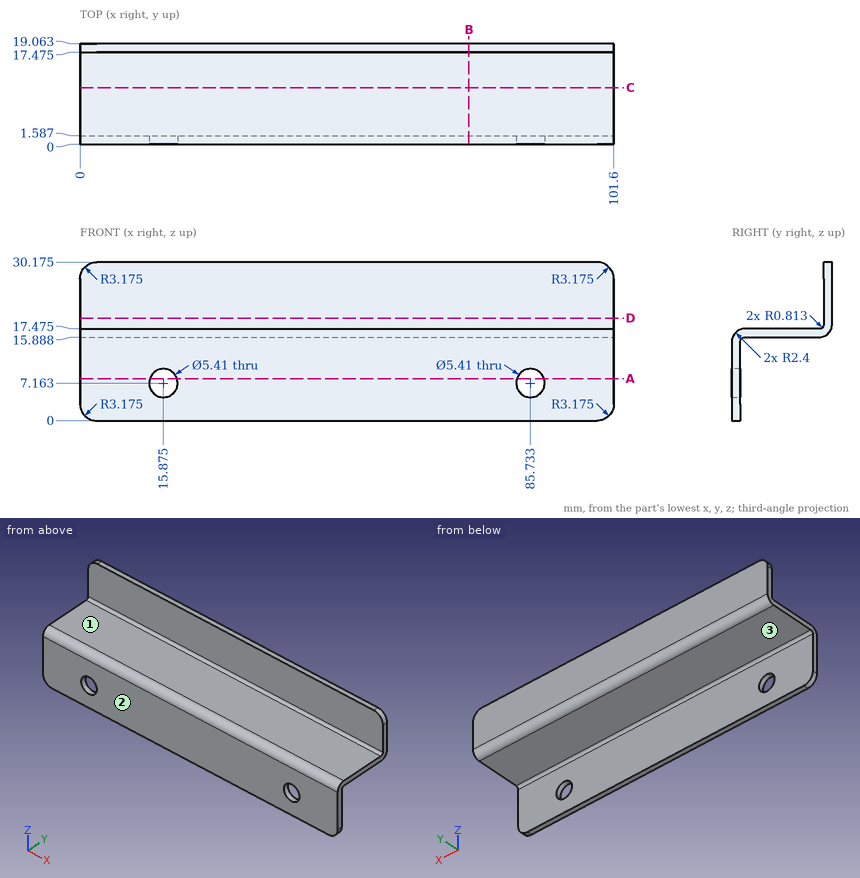
Design review of the part shown in the three views and the two pictorial views. Dimensions are in mm from the part's minimum x, y and z. A direction names the side the tool comes from. Give positions to 0.01 mm unless a question says otherwise; leave off trailing zeros. Loops run counter-clockwise (first coordinate to the right, second up) from the corner with the lowest first, then second, coordinate; pieces in that order, holes last. Notation, with made-up numbers: (30, -20) -> (48, -20) arc R10 cw to (48, -16) -> close; hole circle Ø8 at (-36, -15.5). An arc over 180 degrees is marked (long way). Put each result on its own line as item: value. Start each with the question number.
1. We need section C-C on y = 10.75. State the section outline as (x, z) points (1 decimal), then the cut area to 3 significant figures.
2. Clearance check with flat-ended pins moving along their axes: P1, Ø5, axis at x = 43, z = 14.5, coming from the +Y side; P2, Ø4, axis at y = 2.5, z = 21, coming from the -X side; P3, Ø4.5, axis at x = 57, y = 11.5, coming from the +Z side (1 decimal); P4, Ø12, axis at x = 55, z = 4, coming from the +Y side. State where each tip first meets the part, or that it passes through.
3. We need section D-D on z = 19.5. State the section outline as (x, y) points (1 decimal).
4. For the marked faces 1, 2 and 3, list the 3-axis set-ups (+Z, -Z, +X, -X, +Y, -Y) from which the entire face can be reached by the end or side of a thin tool; tool diameter is ignored.
5. We need section A-A on z = 8. State the section outline as (x, y) points (1 decimal).
6. Wall thickness on probe 1 along Y at (x, z) = (72, 9); probe 2 along Z at (x, y) = (33, 15.25) (1 decimal); probe 3 along Y at (x, z) = (28, 27) (1 decimal): over which ranges is each line inside the solid? List them lowest first.
7. We need section B-B on x = 74. State the section outline as (y, z) points (1 decimal).
Determined:
1. outline: (0, 15.9) -> (101.6, 15.9) -> (101.6, 17.5) -> (0, 17.5) -> close
1. area: 161 mm^2
2. P1: y = 18.69
2. P2: through
2. P3: z = 17.5
2. P4: y = 1.59
3. outline: (0, 17.5) -> (101.6, 17.5) -> (101.6, 19.1) -> (0, 19.1) -> close
4. face 1: +Z, +X, -X, -Y
4. face 2: +Z, -Z, +X, -X, -Y
4. face 3: -Z, +X, -X, +Y
5. outline: (0, 0) -> (13.3, 0) -> (13.3, 1.6) -> (0, 1.6) -> close; (18.4, 0) -> (83.2, 0) -> (83.2, 1.6) -> (18.4, 1.6) -> close; (88.3, 0) -> (101.6, 0) -> (101.6, 1.6) -> (88.3, 1.6) -> close
6. probe 1: 0 to 1.59
6. probe 2: 15.9 to 17.5
6. probe 3: 17.5 to 19.1
7. outline: (0, 0) -> (1.6, 0) -> (1.6, 15.1) arc R0.8 cw to (2.4, 15.9) -> (16.7, 15.9) arc R2.4 ccw to (19.1, 18.3) -> (19.1, 30.2) -> (17.5, 30.2) -> (17.5, 18.3) arc R0.8 cw to (16.7, 17.5) -> (2.4, 17.5) arc R2.4 ccw to (0, 15.1) -> close
